from build123d import *

# Parameters (mm, degrees)
BOSS_EXTRUDE1_DEPTH = 3.175
SKETCH2_W           = 130
SKETCH2_H           = 290
CUT_EXTRUDE1_DEPTH  = 10
SKETCH3_R           = 11.5
SKETCH3_R_2         = 8
SKETCH3_R_3         = 10.25
SKETCH3_R_4         = 12
SKETCH3_R_5         = 12.75
SKETCH3_R_6         = 3
SKETCH3_R_7         = 1.5
SKETCH3_W           = 41
SKETCH3_H           = 98
CUT_EXTRUDE2_DEPTH  = 296.862630114


with BuildPart() as part:
    # Sketch1 → Boss-Extrude1 (new body)
    with BuildSketch(Plane(origin=(0, 0, 0), x_dir=(1, 0, 0), z_dir=(0, 1, 0))):
        with BuildLine():
            Line((-147.955, 238.252), (147.955, 238.252))
            ThreePointArc((147.955, 238.252), (167.352353222, 230.217353222), (175.387, 210.82))
            Line((175.387, 210.82), (175.387, -210.82))
            ThreePointArc((175.387, -210.82), (167.352353222, -230.217353222), (147.955, -238.252))
            Line((147.955, -238.252), (-147.955, -238.252))
            ThreePointArc((-147.955, -238.252), (-167.352353222, -230.217353222), (-175.387, -210.82))
            Line((-175.387, -210.82), (-175.387, 210.82))
            ThreePointArc((-175.387, 210.82), (-167.352353222, 230.217353222), (-147.955, 238.252))
        make_face()
    extrude(amount=BOSS_EXTRUDE1_DEPTH)

    # Sketch2 → Cut-Extrude1 (cut)
    with BuildSketch(Plane(origin=(0, 3.175, 0), x_dir=(1, 0, 0), z_dir=(0, 1, 0))):
        with Locations((110.387, -33.252)):
            Rectangle(SKETCH2_W, SKETCH2_H)
    extrude(amount=-CUT_EXTRUDE1_DEPTH, mode=Mode.SUBTRACT)

    # Sketch3 → Cut-Extrude2 (cut, through all)
    with BuildSketch(Plane(origin=(0, 3.175, 0), x_dir=(1, 0, 0), z_dir=(0, 1, 0))):
        with Locations(Location((-130.387, -193.252, 0), (0, 0, 270))):
            Circle(SKETCH3_R)
        with Locations(Location((-130.387, -133.252, 0), (0, 0, 270))):
            Circle(SKETCH3_R_2)
        with Locations(Location((-130.387, -68.252, 0), (0, 0, 270))):
            Circle(SKETCH3_R_3)
        with Locations(Location((-130.387, -28.252, 0), (0, 0, 270))):
            Circle(SKETCH3_R_4)
        with Locations(Location((-130.387, 11.748, 0), (0, 0, 270))):
            Circle(SKETCH3_R_4)
        with Locations(Location((-130.387, 51.748, 0), (0, 0, 270))):
            Circle(SKETCH3_R_5)
        with Locations(Location((155.387, 218.252, 0), (0, 0, 270))):
            Circle(SKETCH3_R_6)
        with Locations(Location((155.387, -218.252, 0), (0, 0, 270))):
            Circle(SKETCH3_R_6)
        with Locations(Location((-155.387, -218.252, 0), (0, 0, 270))):
            Circle(SKETCH3_R_6)
        with Locations(Location((-155.387, 218.252, 0), (0, 0, 270))):
            Circle(SKETCH3_R_6)
        with Locations(Location((-25.4, 218.252, 0), (0, 0, 270))):
            Circle(SKETCH3_R_7)
        with Locations(Location((25.4, 218.252, 0), (0, 0, 270))):
            Circle(SKETCH3_R_7)
        with Locations(Location((-25.4, -218.252, 0), (0, 0, 270))):
            Circle(SKETCH3_R_7)
        with Locations(Location((25.4, -218.252, 0), (0, 0, 270))):
            Circle(SKETCH3_R_7)
        with Locations((-130.387, 150.748)):
            Rectangle(SKETCH3_W, SKETCH3_H)
    extrude(amount=-CUT_EXTRUDE2_DEPTH, mode=Mode.SUBTRACT)


solid = part.part
Part model, mm, in its own coordinate system. Coordinates: 2 decimals unless noted, no trailing zeros. Write each loop counter-clockwise with the first axis right and the second up, starting at its lowest first coordinate (ties: lowest second). Pieces come first, ordered by that corner, then holes. Notation, with made-up numbers: (69, -2.5) - (78, -2.5) arc R29 cw to (78, 20.5) - close; hole circle Ø8 at (22, -16). An arc over 180 degrees is marked (long way). Put each result on its own line as item: value.
1. Band-saw the part on C-C (y = 1.95). Give the number of separate pieces and of enclosed holes in the cut face, then the cut area to 3 significant figures.
Final values:
separate pieces: 1
enclosed holes: 15
area: 122,000 mm²
2. Flat gauge pins, fed straight in: pin 1 Ø14.5 at (x, z) = (-130.387, -11.748) entering from +Y; pin 2 Ø4 at (x, z) = (25.4, -218.252) entering from -Y. Where does each tip first touch, or does it go through?
Final values:
pin 1: passes through
pin 2: stops at y = 0
3. Band-saw the part on B-B (z = -55). Write the cut outline in (x, y) (3 decimals), then the cut area to 3 significant figures.
Final values:
outline: (-175.387, 0) - (-142.715, 0) - (-142.715, 3.175) - (-175.387, 3.175) - close; (-118.059, 0) - (45.387, 0) - (45.387, 3.175) - (-118.059, 3.175) - close
area: 623 mm²
4. Two-plate mould, pull along X, no slides. Class faces 1 (the cylindrical face through (-167.14, 1.57, 230.43)), 2 (the flat face through (-37, 3.175, -3)), 3 (the cylindrical face through (-120.269, 1.61, 34.703)): +X half, -X half, draft (parallel to the pull), parting line (faces both ways), or undercut.
Final values:
face 1: -X half
face 2: draft
face 3: undercut
5. Probe line 1 along X through (y, z) = (0.85, 28.5); line 2 along X through (y, z) = (1.6, -154.5); line 3 along Z through (x, y) = (154.5, 2.05). List the from-to ranges inside material, lowest first. Write a range as [from, to].
Final values:
line 1: x = [-175.39, -142.38], [-118.39, 45.39]
line 2: x = [-175.39, -150.89], [-109.89, 175.39]
line 3: z = [-237.46, -221.12], [-215.39, -111.75], [178.25, 215.39], [221.12, 237.46]
6. Band-saw the part on A-A (x = 139). Write the cut outline in (y, z) (3 decimals), then the cut area to 3 significant figures.
Final values:
outline: (0, -238.252) - (3.175, -238.252) - (3.175, -111.748) - (0, -111.748) - close; (0, 178.252) - (3.175, 178.252) - (3.175, 238.252) - (0, 238.252) - close
area: 592 mm²
